```python
from build123d import *

# Parameters (mm, degrees)
BOSS_EXTRUDE1_DEPTH        = 3
BOSS_EXTRUDE2_DEPTH        = 10
CHAMFER1_SIZE              = 1.5
LPATTERN1_COUNT            = 3
LPATTERN1_PITCH            = 64
CHAMFER1_OF_LPATTERN1_SIZE = 1.5
MIRROR1_START              = -141
MIRROR1_DEPTH              = 10
MIRROR1_START_2            = -77
MIRROR1_2_DEPTH            = 10
MIRROR1_START_3            = -13
MIRROR1_3_DEPTH            = 10
REVOLVE1_ANGLE             = 18


# Read off the part's stored shape, not the designer's step: Mirror1
with BuildPart() as part:
    # Sketch1 → Boss-Extrude1 (new body)
    with BuildSketch(Plane(origin=(0, 0, 0), x_dir=(1, 0, 0), z_dir=(0, 1, 0))):
        with BuildLine():
            Line((0, 39), (-166, 39))
            Line((-166, 39), (-166, -39))
            Line((-166, -39), (0, -39))
            ThreePointArc((0, -39), (39, 0), (0, 39))
        make_face()
    extrude(amount=BOSS_EXTRUDE1_DEPTH)

    # Sketch3 → Boss-Extrude2 (add)
    with BuildSketch(Plane.ZY.offset(141)):
        Polygon((-34.4, 3), (-34.4, 7.5), (-35.55, 8.65), (-35.55, 9.85), (-34.4, 11), (-30.9, 11), (-30.9, 3), align=None)
    boss_extrude2 = extrude(amount=-BOSS_EXTRUDE2_DEPTH)

    # Chamfer1
    chamfer1_edges = [part.edges().sort_by_distance(p)[0] for p in [
        (-136, 3, -30.9),
    ]]
    chamfer(chamfer1_edges, length=CHAMFER1_SIZE)

    # LPattern1: Boss-Extrude2 ×3
    with Locations(*[(i * LPATTERN1_PITCH, 0, 0) for i in range(1, LPATTERN1_COUNT)]):
        add(boss_extrude2)

    # Chamfer1 of LPattern1
    chamfer1_of_lpattern1_edges = [part.edges().sort_by_distance(p)[0] for p in [
        (-72, 3, -30.9),
        (-8, 3, -30.9),
    ]]
    chamfer(chamfer1_of_lpattern1_edges, length=CHAMFER1_OF_LPATTERN1_SIZE)

    # Mirror1 outline → Mirror1 (add)
    with BuildSketch(Plane.YZ.offset(MIRROR1_START)):
        Polygon((11, 30.9), (11, 34.4), (9.85, 35.55), (8.65, 35.55), (7.5, 34.4), (3, 34.4), (3, 29.4), (4.5, 30.9), align=None)
    extrude(amount=MIRROR1_DEPTH)

    # Mirror1 2 outline → Mirror1 2 (add)
    with BuildSketch(Plane.YZ.offset(MIRROR1_START_2)):
        Polygon((11, 30.9), (11, 34.4), (9.85, 35.55), (8.65, 35.55), (7.5, 34.4), (3, 34.4), (3, 29.4), (4.5, 30.9), align=None)
    extrude(amount=MIRROR1_2_DEPTH)

    # Mirror1 3 outline → Mirror1 3 (add)
    with BuildSketch(Plane.YZ.offset(MIRROR1_START_3)):
        Polygon((11, 30.9), (11, 34.4), (9.85, 35.55), (8.65, 35.55), (7.5, 34.4), (3, 34.4), (3, 29.4), (4.5, 30.9), align=None)
    extrude(amount=MIRROR1_3_DEPTH)

    # Sketch4 → Revolve1 (revolve, symmetric)
    with BuildSketch(Plane.XY) as revolve1_sk:
        Polygon((30.9, 11), (30.9, 3), (34.4, 3), (34.4, 7.5), (35.55, 8.65), (35.55, 9.85), (34.4, 11), align=None)
    revolve(axis=Axis((0, 3, 0), (0, -1, 0)), revolution_arc=REVOLVE1_ANGLE / 2)
    revolve(revolve1_sk.sketch, axis=Axis((0, 3, 0), (0, 1, 0)), revolution_arc=REVOLVE1_ANGLE / 2)


solid = part.part
```
Model file for the job. Use its own axes, mm. A direction names the side the tool comes from. Coordinates: 2 decimals unless noted, no trailing zeros. Order: outer loops, then holes, each group sorted by start corner. A loop starts at its lowest first (then second) coordinate and runs counter-clockwise, first axis right, second up. Notation, with made-up numbers: (10.5, 51) - (60.5, 51) arc R12 cw to (60.5, 60) - close; hole circle Ø2 at (48.5, 20.5). An arc over 180 degrees is marked (long way). Return JSON: item names as keys, results as strings. Group by question number.
1) Mould opens along Z. For faces 1 (the cylindrical face through (38.99, 1.48, 0.86)), 2 (the flat face through (-8, 5, -34.4)), 3 (the flat face through (-77, 7, 33)), 4 (the flat face through (-136, 8, 30.9)) say: released by +Z, released by -Z, zero draft, split by the parting line, or undercut.
2) Flat gauge pins, fed straight in: P1, Ø3, axis at y = 8, z = 33.5, coming from the +X side; P2, Ø0.6, axis at x = -10, y = 9.5, coming from the +Z side; P3, Ø3, axis at x = -79.5, z = 26, coming from the +Y side. Where does each tip first touch, or does it go through?
3) Saw through at C-C, the plane x = -94.5. Write the cut outline in (y, z), plus the area to 3 significant figures.
4) Probe line 1 (X direction, y = 4, z = -34); line 2 (Y direction, x = -53.5, z = 4.5); line 3 (Z direction, x = -74, y = 8.75). List the from-to ranges inside material, lowest first. Write a range as from..to.
5) Saw through at A-A, the plane z = 0. Write the cut outline in (x, y).
6) Saw through at B-B, the plane x = -10.5. Write the cut outline in (y, z).
7) Tool access for faces 5 (the flat face through (-136, 5, 34.4)), 6 (the flat face through (32.27, 7.06, -5.11)), 7 (the flat face through (-8, 8, -30.9)): list every direction of +Z, -Z, +X, -X, +Y, -Y with a clear straight run to the whole face (end or side of a thin tool).
8) Saw through at D-D, the plane z = -26. Write the cut outline in (x, y).
Values found:
{
 "1": {"face 1": "split by the parting line", "face 2": "released by -Z", "face 3": "zero draft", "face 4": "undercut"},
 "2": {"P1": "stops at x = -3", "P2": "stops at z = 35.55", "P3": "stops at y = 3"},
 "3": {"outline": "(0, -39) - (3, -39) - (3, 39) - (0, 39) - close", "area": "234 mm²"},
 "4": {"line 1": "x = -141..-131, -77..-67, -13..-3", "line 2": "y = 0..3", "line 3": "z = -35.55..-30.9, 30.9..35.55"},
 "5": {"outline": "(-166, 0) - (39, 0) - (39, 3) - (34.4, 3) - (34.4, 7.5) - (35.55, 8.65) - (35.55, 9.85) - (34.4, 11) - (30.9, 11) - (30.9, 3) - (-166, 3) - close"},
 "6": {"outline": "(0, -39) - (3, -39) - (3, -34.4) - (7.5, -34.4) - (8.65, -35.55) - (9.85, -35.55) - (11, -34.4) - (11, -30.9) - (4.5, -30.9) - (3, -29.4) - (3, 29.4) - (4.5, 30.9) - (11, 30.9) - (11, 34.4) - (9.85, 35.55) - (8.65, 35.55) - (7.5, 34.4) - (3, 34.4) - (3, 39) - (0, 39) - close"},
 "7": {"face 5": "+Z, +X, -X", "face 6": "-Z, -X, +Y", "face 7": "+X, -X, +Y"},
 "8": {"outline": "(-166, 0) - (29.07, 0) - (29.07, 3) - (-166, 3) - close"}
}
